Geometry: see drawing. Coordinates: mm, zero at the bounding-box minimum. A direction names the side the tool comes from. Coordinates: 2 decimals unless noted, no trailing zeros. Order: outer loops, then holes, each group sorted by start corner. A loop starts at its lowest first (then second) coordinate and runs counter-clockwise, first axis right, second up.
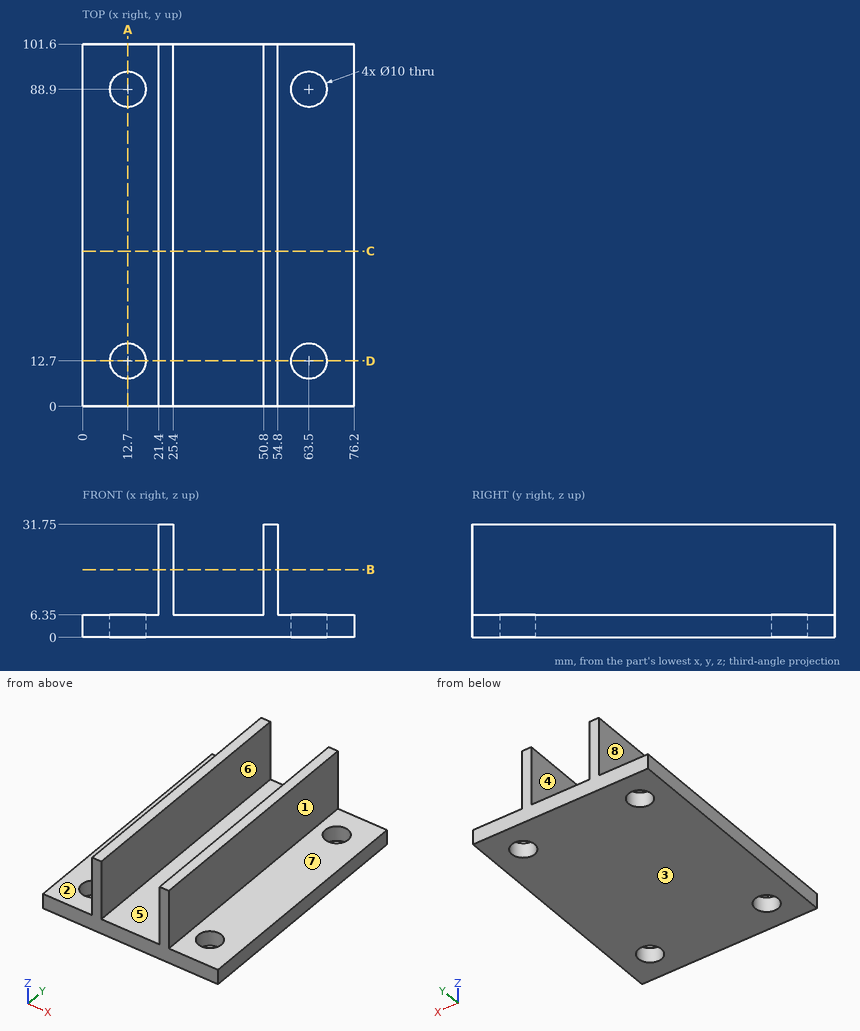
Q1. Section query D-D on y = 12.7. Output: boundary loops of the cut face in (x, z).
Solutions:
outline: (0, 0) - (7.7, 0) - (7.7, 6.35) - (0, 6.35) - close; (17.7, 0) - (58.5, 0) - (58.5, 6.35) - (54.8, 6.35) - (54.8, 31.75) - (50.8, 31.75) - (50.8, 6.35) - (25.4, 6.35) - (25.4, 31.75) - (21.4, 31.75) - (21.4, 6.35) - (17.7, 6.35) - close; (68.5, 0) - (76.2, 0) - (76.2, 6.35) - (68.5, 6.35) - close
Q2. Material intervals for line 1 along Y through (x, z) = (12.7, 1.5); line 2 along X through (y, z) = (42.5, 19.5); line 3 along Z through (x, y) = (65, 24.5), sorted ascending.
Solutions:
line 1: y = 0 to 7.7, 17.7 to 83.9, 93.9 to 101.6
line 2: x = 21.4 to 25.4, 50.8 to 54.8
line 3: z = 0 to 6.35
Q3. Section query A-A on x = 12.7. Output: boundary loops of the cut face in (y, z), plus the area to 3 significant figures.
Solutions:
outline: (0, 0) - (7.7, 0) - (7.7, 6.35) - (0, 6.35) - close; (17.7, 0) - (83.9, 0) - (83.9, 6.35) - (17.7, 6.35) - close; (93.9, 0) - (101.6, 0) - (101.6, 6.35) - (93.9, 6.35) - close
area: 518 mm2
Q4. Pin query (flat end, axial travel): P1, Ø1.5, axis at y = 87.5, z = 6, coming from the -X side; P2, Ø12, axis at y = 72.5, z = 24, coming from the +X side; P3, Ø5, axis at y = 55.5, z = 23, coming from the -X side; P4, Ø13, axis at x = 63.5, y = 88.9, coming from the +Z side. Return the tip coordinate at first contact, or that it passes through.
Solutions:
P1: stops at x = 0
P2: stops at x = 54.8
P3: stops at x = 21.4
P4: stops at z = 6.35
Q5. Set-up query: the marked faces 1, 2, 3 and 4. Return all of +Z, -Z, +X, -X, +Y, -Y with unobstructed straight access to the full face (end or side cutting, diameter ignored); none if empty.
Solutions:
face 1: +Z, +X, +Y, -Y
face 2: +Z, -X, +Y, -Y
face 3: -Z, +X, -X, +Y, -Y
face 4: +Z, +Y, -Y
Q6. Section query B-B on z = 19. Output: boundary loops of the cut face in (x, y), plus the area to 3 significant figures.
Solutions:
outline: (21.4, 0) - (25.4, 0) - (25.4, 101.6) - (21.4, 101.6) - close; (50.8, 0) - (54.8, 0) - (54.8, 101.6) - (50.8, 101.6) - close
area: 813 mm2
Q7. Section query C-C on y = 43.5. Output: boundary loops of the cut face in (x, z), plus the area to 3 significant figures.
Solutions:
outline: (0, 0) - (76.2, 0) - (76.2, 6.35) - (54.8, 6.35) - (54.8, 31.75) - (50.8, 31.75) - (50.8, 6.35) - (25.4, 6.35) - (25.4, 31.75) - (21.4, 31.75) - (21.4, 6.35) - (0, 6.35) - close
area: 687 mm2
Q8. Pull-direction query (X, two-part tool) for the marked faces 5, 6, 7 and 8; classes: pulls with the +X half, pulls with the -X half, needs draft (parallel to the pull), parting line crosses it, or undercut.
Solutions:
face 5: undercut
face 6: undercut
face 7: needs draft
face 8: pulls with the -X half
